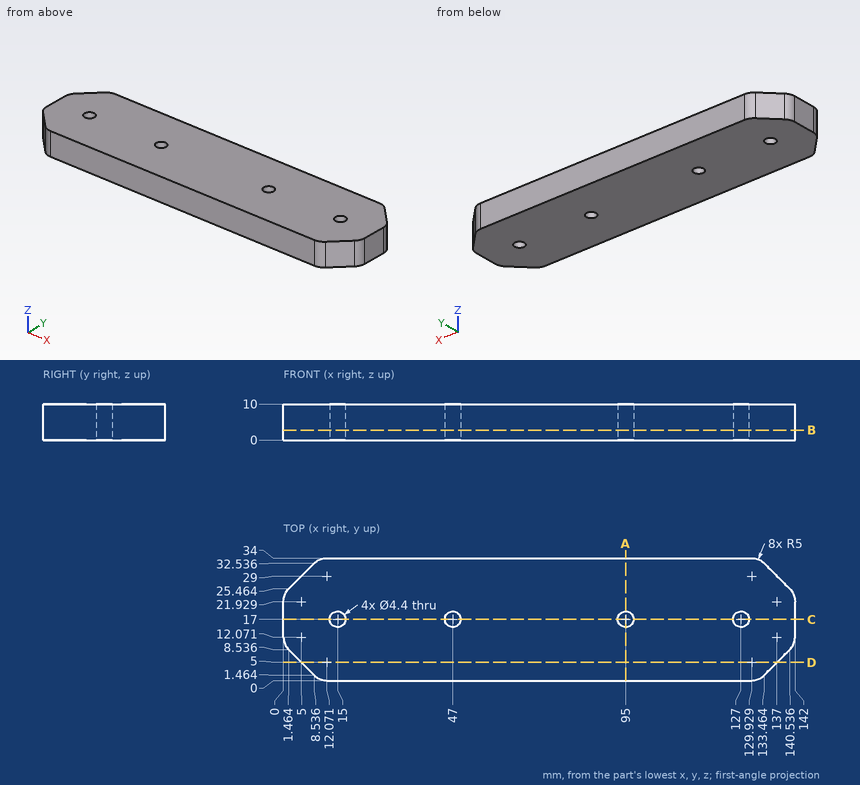
Geometry check sheet. Reference: drawing and pictorial views, mm from the part's lowest x, y, z. Coordinates: 2 decimals unless noted, no trailing zeros. Write each loop counter-clockwise with the first axis right and the second up, starting at its lowest first coordinate (ties: lowest second). Pieces come first, ordered by that corner, then holes. Notation, with made-up numbers: M 69.25,-15 L 123.25,-15 A22 cw 123.25,13 Z; hole C 56,3 d10. An arc over 180 degrees is marked long. Write item = value, one per line. Start each with the question number.
1. Sectioned sample at D-D (y = 5). Record the cut outline in (x, z), then the cut area to 3 significant figures.
2. Sectioned sample at B-B (z = 2.75). Record the cut outline in (x, y) (1 decimal).
3. Sectioned sample at A-A (x = 95). Record the cut outline in (y, z).
4. Sectioned sample at C-C (y = 17). Record the cut outline in (x, z), then the cut area to 3 significant figures.
5. Thickness scan on probe 1 along Y at (x, z) = (47, 4.25); probe 2 along X at (y, z) = (16.5, 8.5); probe 3 along Y at (x, z) = (94.5, 4.25). Record the ranges inside material, lowest first.
The answers:
q1.outline = M 5,0 L 137,0 L 137,10 L 5,10 Z
q1.area = 1,320 mm²
q2.outline = M 0,12.1 A5 ccw 1.5,8.5 L 8.5,1.5 A5 ccw 12.1,0 L 129.9,0 A5 ccw 133.5,1.5 L 140.5,8.5 A5 ccw 142,12.1 L 142,21.9 A5 ccw 140.5,25.5 L 133.5,32.5 A5 ccw 129.9,34 L 12.1,34 A5 ccw 8.5,32.5 L 1.5,25.5 A5 ccw 0,21.9 Z; hole C 15,17 d4.4; hole C 47,17 d4.4; hole C 95,17 d4.4; hole C 127,17 d4.4
q3.outline = M 0,0 L 14.8,0 L 14.8,10 L 0,10 Z; M 19.2,0 L 34,0 L 34,10 L 19.2,10 Z
q4.outline = M 0,0 L 12.8,0 L 12.8,10 L 0,10 Z; M 17.2,0 L 44.8,0 L 44.8,10 L 17.2,10 Z; M 49.2,0 L 92.8,0 L 92.8,10 L 49.2,10 Z; M 97.2,0 L 124.8,0 L 124.8,10 L 97.2,10 Z; M 129.2,0 L 142,0 L 142,10 L 129.2,10 Z
q4.area = 1,240 mm²
q5.probe_1 = 0 to 14.8, 19.2 to 34
q5.probe_2 = 0 to 12.86, 17.14 to 44.86, 49.14 to 92.86, 97.14 to 124.86, 129.14 to 142
q5.probe_3 = 0 to 14.86, 19.14 to 34
